Geometry: see drawing. Coordinates: mm, zero at the bounding-box minimum. Round coordinates to 2 decimals unless told otherwise and drop trailing zeros. Order: outer loops, then holes, each group sorted by start corner. A loop starts at its lowest first (then second) coordinate and runs counter-clockwise, first axis right, second up. Notation, with made-up numbers: M 62,0.25 L 116,0.25 A15 ccw 116,10.25 Z; hole C 56,4.5 d11. An arc over 180 degrees is marked long. Answer in a Markdown table with one row per item. Add a question column.
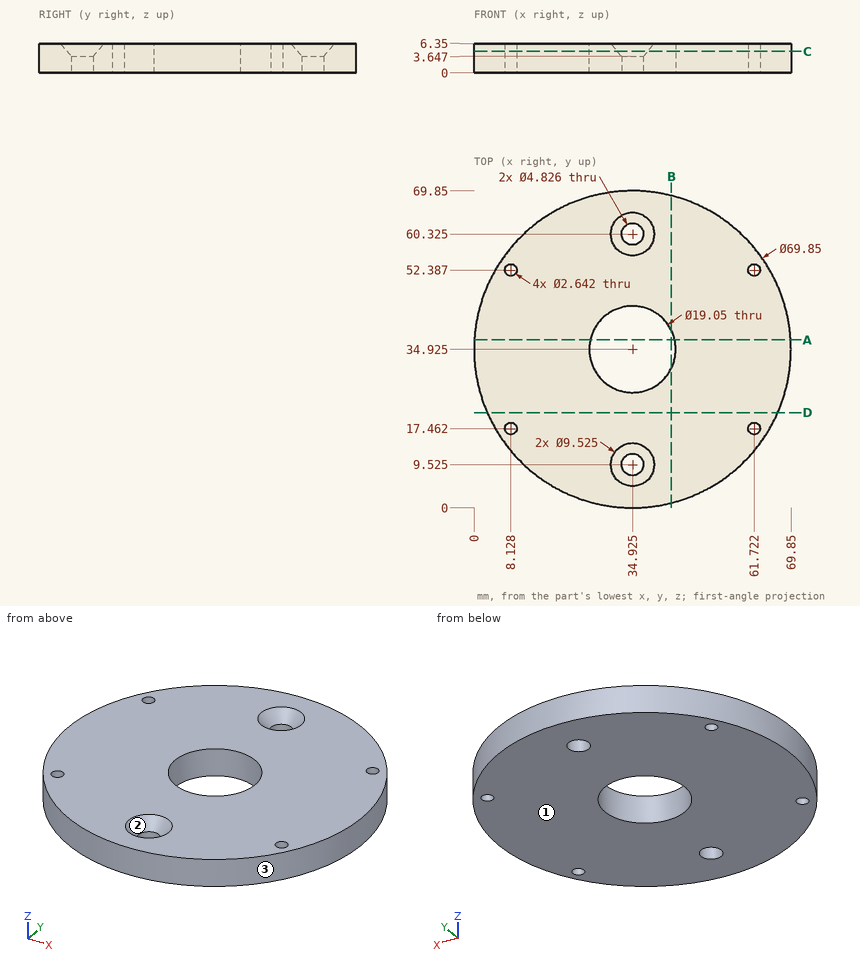
(1) Draft query along X for the marked faces 1, 2 and 3. Return one class per face: +X half, -X half, draft (parallel to the pull), parting line (faces both ways), or undercut.
(2) Pin query (flat end, axial travel): pin 1 (4 mm diameter, centred on x = 34.925, y = 60.325, fed in from +Z); pin 2 (3 mm diameter, centred on y = 54, z = 3, fed in from +X) (1 decimal); pin 3 (1.5 mm diameter, centred on x = 56, z = 1, fed in from -Y) (1 decimal); pin 4 (1.5 mm diameter, centred on x = 48.5, z = 3, fed in from +Y). Return the tip coordinate at first contact, or that it passes through.
(3) Cut plane A-A (y = 37). Return loops of the section in (x, z).
(4) Cut plane D-D (y = 21). Return loops of the section in (x, z).
(5) Cut plane C-C (z = 4.75). Count the separate pieces of the cut face and the enclosed holes in it, and give its area (3 significant figures).
(6) Line query: line 1 (X direction, y = 18, z = 5) (1 decimal); line 2 (X direction, y = 35, z = 5.5); line 3 (Y direction, x = 62.5, z = 4.75) (1 decimal). Output: solid intervals per line, ascending. Write a range as from..to.
(7) Cut plane B-B (x = 43.5). Return loops of the section in (y, z).
Answer list:
| question | item | result |
|---|---|---|
| 1 | face 1 | draft |
| 1 | face 2 | undercut |
| 1 | face 3 | parting line |
| 2 | pin 1 | through |
| 2 | pin 2 | x = 65.1 |
| 2 | pin 3 | y = 6.5 |
| 2 | pin 4 | y = 67.41 |
| 3 | outline | M 0.06,0 L 25.63,0 L 25.63,6.35 L 0.06,6.35 Z; M 44.22,0 L 69.79,0 L 69.79,6.35 L 44.22,6.35 Z |
| 4 | outline | M 2.9,0 L 66.95,0 L 66.95,6.35 L 2.9,6.35 Z |
| 5 | separate pieces | 1 |
| 5 | enclosed holes | 7 |
| 5 | area | 3,450 mm² |
| 6 | line 1 | 4.4..6.9, 9.3..60.5, 62.9..65.5 |
| 6 | line 2 | 0..25.4, 44.45..69.85 |
| 6 | line 3 | 13.5..16.4, 18.5..51.3, 53.5..56.4 |
| 7 | outline | M 1.07,0 L 30.78,0 L 30.78,6.35 L 1.07,6.35 Z; M 39.07,0 L 68.78,0 L 68.78,6.35 L 39.07,6.35 Z |
